Check sheet for the modelled part. Datum: model origin and axes. Units: mm. A direction names the side the tool comes from. Coordinates: 2 decimals unless noted, no trailing zeros. Order: outer loops, then holes, each group sorted by start corner. A loop starts at its lowest first (then second) coordinate and runs counter-clockwise, first axis right, second up. Notation, with made-up numbers: M 41.25,-13.5 L 79.25,-13.5 A13 cw 79.25,-1.5 Z; hole C -3,49 d10. An arc over 180 degrees is marked long. Answer in a Markdown table with one row per item. Add a question column.
from build123d import *

# Parameters (mm, degrees)
SKETCH1_R           = 1.75
SKETCH1_W           = 5
SKETCH1_H           = 5
BOSS_EXTRUDE1_DEPTH = 5
SKETCH2_R           = 3.175
CUT_EXTRUDE1_DEPTH  = 2.5


with BuildPart() as part:
    # Sketch1 → Boss-Extrude1 (new body)
    with BuildSketch(Plane(origin=(0, 0, 0), x_dir=(1, 0, 0), z_dir=(0, 1, 0))):
        Polygon((30, 30), (45, 30), (45, 17.5), (55, 17.5), (55, -17.5), (45, -17.5), (45, -30), (30, -30), (30, -35), (20, -35), (20, -30), (-30, -30), (-30, -35), (-40, -35), (-40, -30), (-45, -30), (-45, 30), (-40, 30), (-40, 35), (-30, 35), (-30, 30), (20, 30), (20, 35), (30, 35), align=None)
        with Locations(Location((37.5, 22.5, 0), (0, 0, 270))):
            Circle(SKETCH1_R, mode=Mode.SUBTRACT)
        with Locations(Location((37.5, -22.5, 0), (0, 0, 270))):
            Circle(SKETCH1_R, mode=Mode.SUBTRACT)
        with Locations(Location((-37.5, 22.5, 0), (0, 0, 270))):
            Circle(SKETCH1_R, mode=Mode.SUBTRACT)
        with Locations(Location((-37.5, -22.5, 0), (0, 0, 270))):
            Circle(SKETCH1_R, mode=Mode.SUBTRACT)
        with Locations((47.5, 10)):
            Rectangle(SKETCH1_W, SKETCH1_H, mode=Mode.SUBTRACT)
        with Locations((47.5, -10)):
            Rectangle(SKETCH1_W, SKETCH1_H, mode=Mode.SUBTRACT)
    extrude(amount=BOSS_EXTRUDE1_DEPTH)

    # Sketch2 → Cut-Extrude1 (cut)
    with BuildSketch(Plane(origin=(0, 5, 0), x_dir=(1, 0, 0), z_dir=(0, 1, 0))):
        with Locations(Location((-37.5, 22.5, 0), (0, 0, 270))):
            Circle(SKETCH2_R)
        with Locations(Location((-37.5, -22.5, 0), (0, 0, 270))):
            Circle(SKETCH2_R)
        with Locations(Location((37.5, 22.5, 0), (0, 0, 270))):
            Circle(SKETCH2_R)
        with Locations(Location((37.5, -22.5, 0), (0, 0, 270))):
            Circle(SKETCH2_R)
    extrude(amount=-CUT_EXTRUDE1_DEPTH, mode=Mode.SUBTRACT)


solid = part.part
1. Section check D-D on y = 3.6. State how many separate pieces and enclosed holes the cut face has, then the cut area to 3 significant figures.
2. Section check A-A on x = 37.5. Enter the section's corners in (y, z) (3 decimals).
3. Scan lines: line 1 (Z direction, x = 37.5, y = 1.15); line 2 (X direction, y = 1.2, z = -22.5); line 3 (X direction, y = 4.15, z = -22.5) (3 decimals). Record each from-to range of solid material in increasing order.
4. Section check B-B on z = 22.5. Enter the section's corners in (x, y) (3 decimals).
5. Section check C-C on x = 48.5. Enter the section's corners in (y, z), then the cut area to 3 significant figures.
6. Set-up check for faces 4 (the flat face through (-5, 2, -30)), 5 (the flat face through (-30, 2, 32)), 6 (the flat face through (45, 2, -10)): record each of +Z, -Z, +X, -X, +Y, -Y from which the full face is reachable in a straight line by a thin tool's end or side.
7. Release check for a two-part mould opening along X. For faces 1 (the flat face through (50, 2, 17.5)), 2 (the flat face through (-40, 2, 33)), 3 (the flat face through (50, 2, -10)) record: released by +X, released by -X, zero draft, split by the parting line, or undercut.
8. Go/stop test with flat-tipped pins: pin 1 Ø5 at (x, z) = (37.5, -22.5) entering from -Y; pin 2 Ø3 at (x, z) = (-38.5, -22) entering from +Y; pin 3 Ø2.5 at (x, y) = (48, 3.5) entering from +Z; pin 4 Ø2.5 at (y, z) = (3.5, 33) entering from -X. Record where each tip stops, or that it passes through.
Result sheet:
| question | item | result |
|---|---|---|
| 1 | separate pieces | 1 |
| 1 | enclosed holes | 6 |
| 1 | area | 5,770 mm^2 |
| 2 | outline | M 0,-30 L 5,-30 L 5,-25.675 L 2.5,-25.675 L 2.5,-24.25 L 0,-24.25 Z; M 0,-20.75 L 2.5,-20.75 L 2.5,-19.325 L 5,-19.325 L 5,19.325 L 2.5,19.325 L 2.5,20.75 L 0,20.75 Z; M 0,24.25 L 2.5,24.25 L 2.5,25.675 L 5,25.675 L 5,30 L 0,30 Z |
| 3 | line 1 | -30 to -24.25, -20.75 to 20.75, 24.25 to 30 |
| 3 | line 2 | -45 to -39.25, -35.75 to 35.75, 39.25 to 45 |
| 3 | line 3 | -45 to -40.675, -34.325 to 34.325, 40.675 to 45 |
| 4 | outline | M -45,0 L -39.25,0 L -39.25,2.5 L -40.675,2.5 L -40.675,5 L -45,5 Z; M -35.75,0 L 35.75,0 L 35.75,2.5 L 34.325,2.5 L 34.325,5 L -34.325,5 L -34.325,2.5 L -35.75,2.5 Z; M 39.25,0 L 45,0 L 45,5 L 40.675,5 L 40.675,2.5 L 39.25,2.5 Z |
| 5 | outline | M 0,-17.5 L 5,-17.5 L 5,-12.5 L 0,-12.5 Z; M 0,-7.5 L 5,-7.5 L 5,7.5 L 0,7.5 Z; M 0,12.5 L 5,12.5 L 5,17.5 L 0,17.5 Z |
| 5 | area | 125 mm^2 |
| 6 | face 4 | -Z, +Y, -Y |
| 6 | face 5 | +Z, +Y, -Y |
| 6 | face 6 | +Y, -Y |
| 7 | face 1 | zero draft |
| 7 | face 2 | released by -X |
| 7 | face 3 | undercut |
| 8 | pin 1 | y = 0 |
| 8 | pin 2 | y = 2.5 |
| 8 | pin 3 | z = 17.5 |
| 8 | pin 4 | x = -40 |
